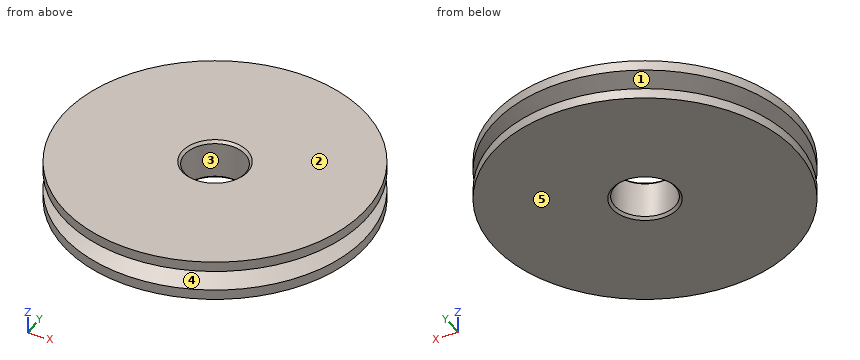
```python
from build123d import *

# Parameters (mm, degrees)
SKETCH1_R      = 47.625
SKETCH1_R_2    = 9.525
EXTRUDE1_DEPTH = 6.35
CHAMFER1_SIZE  = 0.79375


with BuildPart() as part:
    # Sketch1 → Extrude1 (new, symmetric)
    with BuildSketch(Plane.XY):
        Circle(SKETCH1_R)
        Circle(SKETCH1_R_2, mode=Mode.SUBTRACT)
    extrude(amount=EXTRUDE1_DEPTH, both=True)

    # Chamfer1
    chamfer1_edges = [part.edges().sort_by_distance(p)[0] for p in [
        (-9.525, 0, -6.35),
        (-9.525, 0, 6.35),
    ]]
    chamfer(chamfer1_edges, length=CHAMFER1_SIZE)

    # Sketch2 → Cut-Revolve1 (revolve, cut)
    with BuildSketch(Plane(origin=(0, 0, 0), x_dir=(0, 0, -1), z_dir=(1, 0, 0)), mode=Mode.PRIVATE) as cut_revolve1_sk:
        Polygon((-3.175, 47.625), (3.175, 47.625), (0.863789012, 41.275), (-0.863789012, 41.275), align=None)
    revolve(cut_revolve1_sk.sketch.rotate(Axis((0, 0, 6.35), (0, 0, -1)), 180), axis=Axis((0, 0, 6.35), (0, 0, -1)), mode=Mode.SUBTRACT)


solid = part.part
```
Geometry check sheet. Reference: the model listing, model coordinates, mm. Face numbers are marked on the shaded views. A direction names the side the tool comes from. Round coordinates to 2 decimals unless told otherwise and drop trailing zeros. Order: outer loops, then holes, each group sorted by start corner. A loop starts at its lowest first (then second) coordinate and runs counter-clockwise, first axis right, second up. Notation, with made-up numbers: (53, -25) - (72, -25) arc R34 cw to (72, 6) - close; hole circle Ø10 at (83.5, 66.25). An arc over 180 degrees is marked (long way). Use a Markdown table: item, result. Add a question column.
(1) Release check for a two-part mould opening along X. For the marked faces 3, 4 and 5 record: pulls with the +X half, pulls with the -X half, needs draft (parallel to the pull), parting line crosses it, or undercut.
(2) Material ranges on line 1 along Y through (x, z) = (0, 3.25) (3 decimals); line 2 along Z through (x, y) = (-36.5, -24); line 3 along Z through (x, y) = (-40, -14), recorded low to high. Write a range as [from, to].
(3) Tool access check on the marked faces 1 and 2. Record the directions out of +Z, -Z, +X, -X, +Y, -Y that give a thin tool (end or side, any length) a straight path to the whole face; none if there is none.
(4) Sectioned sample at A-A, the plane x = 0. Enter the section's corners in (y, z) (3 decimals), and give its area (3 significant figures).
(5) Depth check by flat-ended pin: pin 1 (1.5 mm diameter, centred on x = -3.5, z = -3.5, fed in from +Y). Enter the tip coordinate at first touch or a pass-through.
Answers below:
| question | item | result |
|---|---|---|
| 1 | face 3 | undercut |
| 1 | face 4 | parting line crosses it |
| 1 | face 5 | needs draft |
| 2 | line 1 | [-47.625, -9.525], [9.525, 47.625] |
| 2 | line 2 | [-6.35, -1.74], [1.74, 6.35] |
| 2 | line 3 | [-6.35, -1.27], [1.27, 6.35] |
| 3 | face 1 | none |
| 3 | face 2 | +Z, +X, -X, +Y, -Y |
| 4 | outline | (-47.625, -6.35) - (-10.319, -6.35) - (-9.525, -5.556) - (-9.525, 5.556) - (-10.319, 6.35) - (-47.625, 6.35) - (-47.625, 3.175) - (-41.275, 0.864) - (-41.275, -0.864) - (-47.625, -3.175) - close; (9.525, -5.556) - (10.319, -6.35) - (47.625, -6.35) - (47.625, -3.175) - (41.275, -0.864) - (41.275, 0.864) - (47.625, 3.175) - (47.625, 6.35) - (10.319, 6.35) - (9.525, 5.556) - close |
| 4 | area | 915 mm² |
| 5 | pin 1 | y = 47.55 |
